Verification items for the finished model (mm, model axes). A direction names the side the tool comes from. Coordinates: 2 decimals unless noted, no trailing zeros. Loops run counter-clockwise (first coordinate to the right, second up) from the corner with the lowest first, then second, coordinate; pieces in that order, holes last. Notation, with made-up numbers: (83, 23) -> (105, 23) arc R23 cw to (105, 55) -> close; hole circle Ø2 at (-29.5, 45.5). An arc over 180 degrees is marked (long way). Answer as a JSON object with one key per item and string values. Group by question number.
Q1. Set-up check for faces 4 (the flat face through (-249, 0, -6)), 5 (the flat face through (-578, 9, -12.7)): record each of +Z, -Z, +X, -X, +Y, -Y from which the full face is reachable in a straight line by a thin tool's end or side.
Q2. Scan lines: L1, parallel to Z at x = 0, y = 5.5; L2, parallel to Z at x = -571, y = 17.25; L3, parallel to X at y = 9, z = 0. Record each from-to range of solid material in increasing order.
Q3. Gauge pin test, flat ends, axial feed: pin 1 Ø5.5 at (y, z) = (12, -1) entering from -X; pin 2 Ø8 at (y, z) = (14.5, -77.5) entering from +X; pin 3 Ø5 at (y, z) = (9.5, 8.5) entering from +X. Record the tip position at first contact, or that the pin passes through.
Q4. Cross-section at B-B on z = -79. Record the boundary of the cut face in (x, y).
Q5. Cross-section at A-A on y = 4.5. Give the number of separate pieces and of enclosed holes in the cut face, and give its area (3 significant figures).
Q6. Release check for a two-part mould opening along Z. For faces 1 (the flat face through (-508.927, 9, 0)), 2 (the flat face through (-339, 9, -74)), 3 (the cylindrical face through (-615.945, 9.392, 0.419)) record: released by +Z, released by -Z, zero draft, split by the parting line, or undercut.
Q7. Cross-section at C-C on x = -421. Record the boundary of the cut face in (y, z), and give its area (3 significant figures).
```python
from build123d import *

# Parameters (mm, degrees)
SKETCH1_R           = 12.7
BOSS_EXTRUDE1_DEPTH = 19.05


with BuildPart() as part:
    # Sketch1 → Boss-Extrude1 (new body)
    with BuildSketch(Plane(origin=(0, 0, 0), x_dir=(1, 0, 0), z_dir=(0, 1, 0))):
        with BuildLine():
            Line((0, -19.05), (-558.8, -19.05))
            Line((-558.8, -19.05), (-596.9, -19.05))
            ThreePointArc((-596.9, -19.05), (-615.95, 0), (-596.9, 19.05))
            Line((-596.9, 19.05), (-561.926882891, 19.05))
            ThreePointArc((-561.926882891, 19.05), (-558.823427993, 19.24030806), (-555.766478015, 19.808380496))
            Line((-555.766478015, 19.808380496), (-116.049044826, 129.737738793))
            ThreePointArc((-116.049044826, 129.737738793), (-102.738548138, 129.468976879), (-91.392360136, 122.504382644))
            Line((-91.392360136, 122.504382644), (0, 25.4))
            Line((0, 25.4), (16.653962733, 7.705164597))
            ThreePointArc((16.653962733, 7.705164597), (19.666677712, -9.47154715), (5.093787849, -19.05))
            Line((5.093787849, -19.05), (0, -19.05))
        make_face()
        Circle(SKETCH1_R, mode=Mode.SUBTRACT)
        with BuildLine():
            Line((-596.9, -12.7), (-558.8, -12.7))
            ThreePointArc((-558.8, -12.7), (-551.700484171, -10.530283709), (-547.026784902, -4.7625))
            Line((-547.026784902, -4.7625), (-521.626784902, -4.7625))
            Line((-521.626784902, -4.7625), (-521.626784902, -9.525))
            Line((-521.626784902, -9.525), (-508.926784902, -9.525))
            Line((-508.926784902, -9.525), (-508.926784902, 9.525))
            Line((-508.926784902, 9.525), (-521.626784902, 9.525))
            Line((-521.626784902, 9.525), (-521.626784902, 4.7625))
            Line((-521.626784902, 4.7625), (-547.026784902, 4.7625))
            ThreePointArc((-547.026784902, 4.7625), (-551.700484171, 10.530283709), (-558.8, 12.7))
            Line((-558.8, 12.7), (-596.9, 12.7))
            ThreePointArc((-596.9, 12.7), (-609.6, 0), (-596.9, -12.7))
        make_face(mode=Mode.SUBTRACT)
        with BuildLine():
            Line((-401.666524357, 25.115607314), (-139.08105489, 90.761974681))
            ThreePointArc((-139.08105489, 90.761974681), (-134.089618632, 90.661188963), (-129.834798131, 88.049466125))
            Line((-129.834798131, 88.049466125), (-68.049981786, 22.403098758))
            ThreePointArc((-68.049981786, 22.403098758), (-66.242352798, 12.09707171), (-74.986086716, 6.35))
            Line((-74.986086716, 6.35), (-399.356372528, 6.35))
            ThreePointArc((-399.356372528, 6.35), (-408.810007006, 14.711204413), (-401.666524357, 25.115607314))
        make_face(mode=Mode.SUBTRACT)
    extrude(amount=BOSS_EXTRUDE1_DEPTH)


solid = part.part
```
Computed values:
{
 "1": {"face 4": "+Z, -Z, +X, -X, -Y", "face 5": "+Y, -Y"},
 "2": {"L1": "z = -25.4 to -12.7, 12.7 to 19.05", "L2": "z = -19.05 to -12.7, 12.7 to 19.05", "L3": "x = -615.95 to -609.6, -508.93 to -12.7, 12.7 to 20.65"},
 "3": {"pin 1": "stops at x = -615.95", "pin 2": "stops at x = -45.27", "pin 3": "stops at x = 20.72"},
 "4": {"outline": "(-319, 0) -> (-186.13, 0) -> (-186.13, 19.05) -> (-319, 19.05) -> close; (-121.32, 0) -> (-50.45, 0) -> (-50.45, 19.05) -> (-121.32, 19.05) -> close"},
 "5": {"separate pieces": "1", "enclosed holes": "3", "area": "36,300 mm²"},
 "6": {"face 1": "undercut", "face 2": "released by -Z", "face 3": "split by the parting line"},
 "7": {"outline": "(0, -53.5) -> (19.05, -53.5) -> (19.05, 19.05) -> (0, 19.05) -> close", "area": "1,380 mm²"}
}
